Could you check a few things on this model? Use its own coordinates, in mm. A direction names the side the tool comes from. Give positions to 0.01 mm unless a question says otherwise; leave off trailing zeros. Loops run counter-clockwise (first coordinate to the right, second up) from the corner with the lowest first, then second, coordinate; pieces in that order, holes last.
1. For P1, Ø4, axis at y = 2.5, z = 3.5, coming from the -X side; P2, Ø4, axis at x = 25.5, z = 3.5, coming from the -Y side; P3, Ø3.5, axis at y = -2.5, z = 5, coming from the +X side; P4, Ø2.5, axis at x = -25.5, z = 3.5, coming from the +Y side, each with a flat end and sliding along its axis, tell me the tip position at first contact or that it passes through.
2. I need wall thicknesses on line 1 along Y through (x, z) = (0, 3.1); line 2 along X through (y, z) = (0, 5.4); line 3 along Z through (x, y) = (11, 4.5). Which ranges of each line are inside material? Lowest first, please.
3. Imagine slicing it at C-C (y = -1). List the corners of the cut face in (x, z) for me.
4. Thinking about a two-plate mould opening in Z: for faces 5 (the cylindrical face through (25.292, -11.479, 1.914)), 6 (the cylindrical face through (11.437, 11.189, 3.549)), 7 (the flat face through (-6, -8, 0)), 8 (the flat face through (-3, -8, 2)), which applies, +Z half, -Z half, draft (parallel to the pull), parting line (faces both ways), or undercut?
5. For faces 1 (the flat face through (23, -10, 3)), 2 (the flat face through (19.5, -15, 4)), 3 (the flat face through (-23, -13, 3)), 4 (the flat face through (-16, -3, 3)), which set-ups out of +Z, -Z, +X, -X, +Y, -Y let a thin tool reach every point of the face, with its end or its side?
6. Imagine slicing it at B-B (x = -25.5). List the corners of the cut face in (y, z) for me, plus the area to 3 significant figures.
7. Imagine slicing it at A-A (z = 3.5). Count the separate pieces of the cut face and the enclosed holes in it, plus the area to 3 significant figures.
8. Imagine slicing it at D-D (x = -9). List the corners of the cut face in (y, z) for me.
Autodesk Inventor part; units mm, degrees
ref_plane "YZ Plane" through (0, 0, 0) normal (1, 0, 0) x (0, 1, 0)
ref_plane "XZ Plane" through (0, 0, 0) normal (0, 1, 0) x (-1, 0, 0)
ref_plane "XY Plane" through (0, 0, 0) normal (0, 0, 1) x (1, 0, 0)
sketch "Skizze1" plane through (0, 0, 0) normal (0, 0, 1) x (1, 0, 0)
  line L0 (0, 22.4) -> (0, -22.4)
  line L1 (-22.4, 0) -> (22.4, 0)
  line L2 (-16, 16) -> (16, 16)
  line L3 (16, 16) -> (16, -16)
  line L4 (16, -16) -> (-16, -16)
  line L5 (-16, -16) -> (-16, 16)
  circle A0 centre (0, 0) radius 12.1
  dimension "d0" = 32
  dimension "d1" = 32
  dimension "d2" = 24.2
extrude "Extrusion1" add sketch "Skizze1" along normal blind 7 contours L2 L3 L1 A0 L0 | L0 A0 L1 L5 L2 | L1 L3 L4 L0 A0 | A0 L0 L4 L5 L1
sketch "Skizze2" plane through (16, -16, 0) normal (1, 0, 0) x (0, 0, -1)
  line L0 (-7, 32) -> (-7, 0)
  line L1 (0, 32) -> (0, 0)
  line L2 (-7, 0) -> (0, 0)
  line L3 (0, 0) -> (0, 6)
  line L4 (0, 6) -> (-7, 6)
  line L5 (-7, 6) -> (-7, 0)
  line L6 (0, 3) -> (-7, 3)
  point P0 (0, 16)
  point P1 (-7, 6)
  point P2 (0, 3)
  dimension "d5" = 6
sketch "Skizze3" plane through (-16, -16, 0) normal (-1, 0, 0) x (0, 0, 1)
  line L0 (7, 32) -> (7, 0)
  line L1 (0, 32) -> (0, 0)
  line L2 (7, 0) -> (0, 0)
  line L3 (0, 0) -> (0, 6)
  line L4 (0, 6) -> (7, 6)
  line L5 (7, 6) -> (7, 0)
  line L6 (0, 3) -> (7, 3)
  point P0 (0, 16)
  point P1 (7, 6)
  point P2 (0, 3)
  point P3 (7, 3)
  dimension "d6" = 6
sketch "Skizze4" plane through (0, 0, 0) normal (0, 0, -1) x (-1, 0, 0)
  circle A0 centre (0, 0) radius 12.1
  circle A1 centre (0, 0) radius 12.1
  circle A2 centre (0, 0) radius 8.25
  dimension "d11" = 24.2
  dimension "d12" = 16.5
extrude "Extrusion4" add sketch "Skizze4" against normal blind 2
fillet "Rundung1" radius 16 2 edges at (16, 16, 3.5) (-16, 16, 3.5)
extrude "Extrusion6" add sketch "Skizze3" along normal blind 13 contours L0 L6 L1 L4
extrude "Extrusion7" add sketch "Skizze2" along normal blind 13 contours L4 L1 L6 L0
sketch "Skizze6" plane through (16, -10, 7) normal (0, 1, 0) x (1, 0, 0)
  circle A0 centre (9.5, 3.5) radius 1.6
  line L0 (0, 7) -> (13, 7)
  line L1 (13, 7) -> (13, 0)
  circle A1 centre (-41.5, 3.5) radius 1.6
  line L2 (-45, 0) -> (-45, 7)
  line L3 (-32, 7) -> (-45, 7)
  point P0 (-16, 7)
  dimension "d29" = 3.2
  dimension "d30" = 3.5
  dimension "d31" = 3.5
  dimension "d32" = 3.2
  dimension "d33" = 3.5
  dimension "d34" = 3.5
extrude "Extrusion8" cut sketch "Skizze6" against normal up to surface (3 mm away)
sketch "Skizze7" plane through (16, -16, 7) normal (1, 0, 0) x (0, 0, -1)
  line L0 (7, 0) -> (0, 0)
  line L1 (0, 3) -> (0, 0)
  line L2 (7, 0) -> (0, 0)
  line L3 (0, 0) -> (0, 3)
  line L4 (0, 3) -> (7, 3)
  line L5 (7, 3) -> (7, 0)
  point P0 (7, 16)
extrude "Extrusion9" add sketch "Skizze7" along normal blind 3.5
sketch "Skizze8" plane through (-16, -16, 0) normal (-1, 0, 0) x (0, 0, 1)
  line L0 (0, 0) -> (7, 0)
  line L1 (0, 0) -> (0, 3)
  line L2 (7, 0) -> (0, 0)
  line L3 (0, 0) -> (0, 3)
  line L4 (0, 3) -> (7, 3)
  line L5 (7, 3) -> (7, 0)
  point P0 (0, 16)
extrude "Extrusion10" add sketch "Skizze8" along normal blind 3.5
fillet "Rundung3" radius 3.5 2 edges at (16, -10, 3.5) (-16, -10, 3.5)
sketch "Skizze9" plane through (19.5, -16, 0) normal (0, -1, 0) x (1, 0, 0)
  line L0 (0, 7) -> (-39, 7)
  line L1 (0, 0) -> (9.5, 0)
  line L2 (-39, 7) -> (0, 7)
  line L3 (0, 7) -> (0, 0)
  line L4 (0, 0) -> (-39, 0)
  line L5 (-39, 0) -> (-39, 7)
  point P0 (-19.5, 0)
extrude "Extrusion11" add sketch "Skizze9" along normal blind 1.5
properties part number "_3D-Druck"
Derived:
1. P1: stops at x = -15.99
1. P2: stops at y = -13
1. P3: stops at x = 16
1. P4: passes through
2. line 1: y = -17.5 to -12.1, 12.1 to 16
2. line 2: x = -16 to -12.1, 12.1 to 16
2. line 3: z = 0 to 2
3. outline: (-16, 0) - (-8.19, 0) - (-8.19, 2) - (-12.06, 2) - (-12.06, 7) - (-16, 7) - close; (8.19, 0) - (16, 0) - (16, 7) - (12.06, 7) - (12.06, 2) - (8.19, 2) - close
4. face 5: undercut
4. face 6: draft
4. face 7: -Z half
4. face 8: +Z half
5. face 1: +Z, -Z, +X, +Y
5. face 2: +Z, -Z, +X, -Y
5. face 3: +Z, -Z, -X, -Y
5. face 4: +Z, -Z, -X, +Y
6. outline: (-13, 0) - (-10, 0) - (-10, 1.9) - (-13, 1.9) - close; (-13, 5.1) - (-10, 5.1) - (-10, 7) - (-13, 7) - close
6. area: 11.4 mm2
7. separate pieces: 3
7. enclosed holes: 1
7. area: 598 mm2
8. outline: (-17.5, 0) - (13.23, 0) - (13.23, 7) - (8.09, 7) - (8.09, 2) - (-8.09, 2) - (-8.09, 7) - (-17.5, 7) - close
